Can you work these out from the model? Positions are in its coordinate system, mm. A direction names the side the tool comes from. Give positions to 0.01 mm unless a question says otherwise; leave off trailing zeros. Write each loop counter-clockwise with the first axis right and the second up, starting at its lowest first coordinate (ties: lowest second). Pieces come first, ordered by that corner, then holes.
from build123d import *

# Parameters (mm, degrees)
SKETCH_1_W      = 40
SKETCH_1_H      = 70
EXTRUDE_3_DEPTH = 50
SKETCH_6_W      = 30
SKETCH_6_H      = 30
EXTRUDE_6_DEPTH = 30


with BuildPart() as part:
    # Эскиз1 → Бобышка-Вытянуть3 (new body)
    with BuildSketch(Plane.XY):
        with BuildLine():
            Line((-100, -215), (-200, -215))
            Line((-200, -215), (-200, -165))
            add(Edge.make_bspline(
                [(-200, 165), (-56.658015908, 0), (-200, -165)],
                knots=[0, 0, 0, 1, 1, 1], degree=2))
            Line((-200, 165), (-200, 215))
            Line((-200, 215), (0, 215))
            Line((0, 215), (200, 215))
            Line((200, 215), (200, 165))
            add(Edge.make_bspline(
                [(200, 165), (56.658015908, 0), (200, -165)],
                knots=[0, 0, 0, 1, 1, 1], degree=2))
            Line((200, -165), (200, -215))
            Line((200, -215), (100, -215))
            ThreePointArc((100, -215), (0, -115), (-100, -215))
        make_face()
        with Locations((0, 95)):
            Rectangle(SKETCH_1_W, SKETCH_1_H, mode=Mode.SUBTRACT)
    extrude(amount=EXTRUDE_3_DEPTH)

    # Эскиз6 → Бобышка-Вытянуть6 (add)
    with BuildSketch(Plane(origin=(0, 215, 0), x_dir=(1, 0, 0), z_dir=(0, 1, 0))):
        with Locations((-175, -25)):
            Rectangle(SKETCH_6_W, SKETCH_6_H)
        with Locations((-125, -25)):
            Rectangle(SKETCH_6_W, SKETCH_6_H)
        with Locations((-75, -25)):
            Rectangle(SKETCH_6_W, SKETCH_6_H)
        with Locations((-25, -25)):
            Rectangle(SKETCH_6_W, SKETCH_6_H)
        with Locations((25, -25)):
            Rectangle(SKETCH_6_W, SKETCH_6_H)
        with Locations((75, -25)):
            Rectangle(SKETCH_6_W, SKETCH_6_H)
        with Locations((125, -25)):
            Rectangle(SKETCH_6_W, SKETCH_6_H)
        with Locations((175, -25)):
            Rectangle(SKETCH_6_W, SKETCH_6_H)
    extrude(amount=EXTRUDE_6_DEPTH)


solid = part.part
(1) For faces 4 (the face through (75, 230, 10)), 5 (the face through (-125, 230, 40)), 6 (the face through (0, 60, 25)), 7 (the face through (-160, 230, 25)), which set-ups out of +Z, -Z, +X, -X, +Y, -Y let a thin tool reach every point of the face, with its end or its side?
Returned:
face 4: -Z, +X, -X, +Y
face 5: +Z, +X, -X, +Y
face 6: +Z, -Z
face 7: +Z, -Z, +Y
(2) If I drill on L1, parallel to Y at x = 1.5, z = 27; L2, parallel to X at y = 76, z = 7.5; L3, parallel to X at y = 117, z = 25, over which ranges is the centre line in solid material (lowest first)?
Returned:
L1: y = -115.01 to 60, 130 to 215
L2: x = -143.53 to -20, 20 to 143.53
L3: x = -164.37 to -20, 20 to 164.37
(3) Imagine slicing it at B-B, the plane x = -53. Write out the boundary of the cut face in (y, z).
Returned:
outline: (-130.2, 0) - (215, 0) - (215, 50) - (-130.2, 50) - close
(4) Will these pins go through, and if not, where does the flat tip stop? P1, Ø4, axis at x = -33.5, z = 7.5, coming from the +Y side; P2, Ø9, axis at x = -119.5, y = 230.5, coming from the +Z side; P3, Ø9, axis at x = -30, y = 229, coming from the -Z side.
Returned:
P1: stops at y = 215
P2: stops at z = 40
P3: stops at z = 10
(5) Imagine slicing it at A-A, the plane x = 0. Write out the boundary of the cut face in (y, z), plus the area to 3 significant figures.
Returned:
outline: (-115, 0) - (60, 0) - (60, 50) - (-115, 50) - close; (130, 0) - (215, 0) - (215, 50) - (130, 50) - close
area: 13,000 mm2
(6) If we mould it in two halves opening along Y, with no side actions, what happens to faces 1 (the face through (-20, 95, 25)), 2 (the face through (-60, 230, 25)), 3 (the face through (125, 245, 25))? For each: +Y half, -Y half, draft (parallel to the pull), parting line (faces both ways), or undercut.
Returned:
face 1: undercut
face 2: draft
face 3: +Y half
